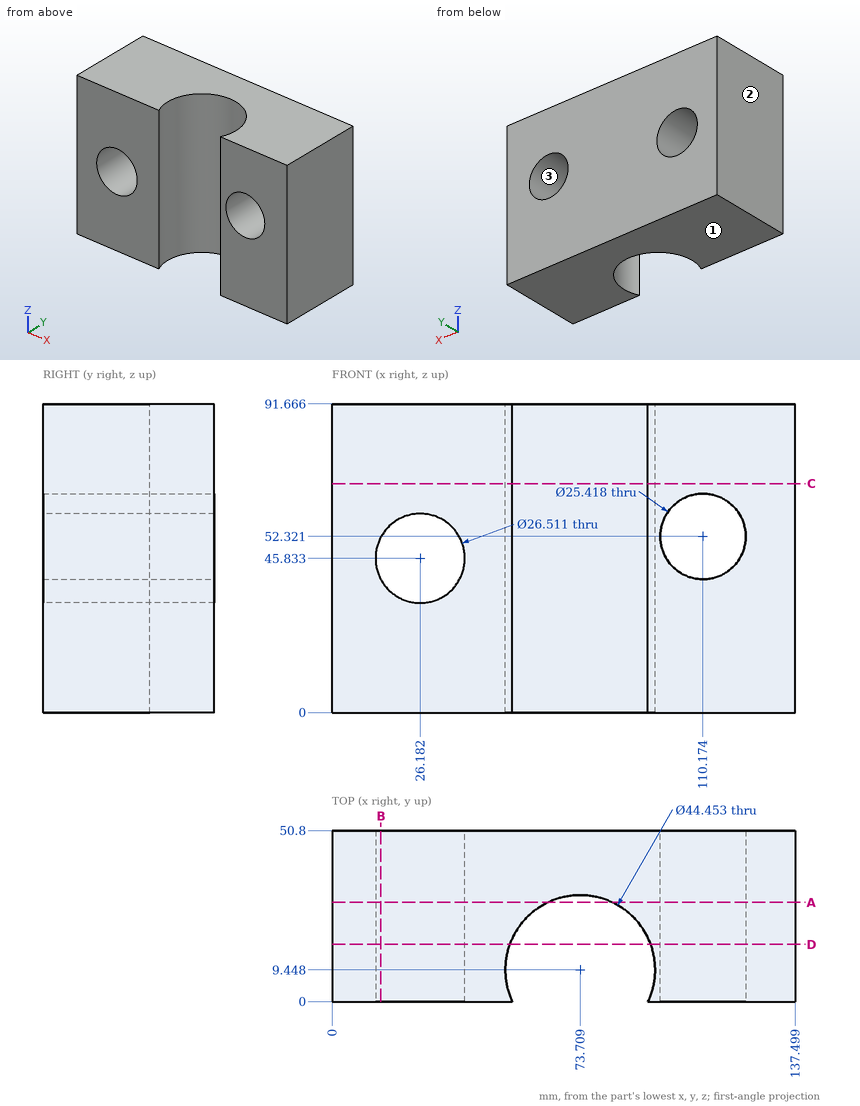
Study the drawing (mm; zero at the part's minimum x, y, z) and answer. Coordinates: 2 decimals unless noted, no trailing zeros. Loops run counter-clockwise (first coordinate to the right, second up) from the corner with the lowest first, then second, coordinate; pieces in that order, holes last. Notation, with made-up numbers: (18, 44.25) -> (30, 44.25) arc R27 ccw to (30, 77.25) -> close; hole circle Ø7 at (87.25, 89). An arc over 180 degrees is marked (long way). Answer in a Markdown table with one row per item. Add a question column.
1. The part is cut by section C-C, the plane z = 68. Write down the section's boundary in (x, y), then the cut area to 3 significant figures.
2. The part is cut by section A-A, the plane y = 29.5. Write down the section's boundary in (x, z) (1 decimal).
3. Flat-ended cylindrical pins translate along their axes: P1, Ø8, axis at x = 89.5, y = 33.5, coming from the -Z side; P2, Ø1, axis at x = 77.5, z = 80.5, coming from the -Y side; P3, Ø21, axis at x = 26.18, z = 45.83, coming from the +Y side; P4, Ø3, axis at x = 83.5, z = 29.5, coming from the -Y side (1 decimal). Find the tip coordinate at first contact, or state that the pin passes through.
4. Consider line 1 (X direction, y = 7, z = 62.5) (1 decimal); line 2 (Z direction, x = 104, y = 18) (1 decimal); line 3 (Z direction, x = 115.5, y = 13) (1 decimal). Determine where each line is inside the solid, lowest interval first. Write a range as [from, to].
5. The part is cut by section D-D, the plane y = 17. Write down the section's boundary in (x, z) (1 decimal).
6. The part is cut by section B-B, the plane x = 14.5. Write down the section's boundary in (y, z) (1 decimal), then the cut area to 3 significant figures.
7. Determine the mould class of the marked faces 1, 2 and 3 for opening direction Z: +Z half, -Z half, draft (parallel to the pull), parting line (faces both ways), or undercut.
Answer below:
| question | item | result |
|---|---|---|
| 1 | outline | (0, 0) -> (53.59, 0) arc R22.23 cw (long way) to (93.83, 0) -> (137.5, 0) -> (137.5, 50.8) -> (0, 50.8) -> close |
| 1 | area | 5,800 mm2 |
| 2 | outline | (0, 0) -> (64.1, 0) -> (64.1, 91.7) -> (0, 91.7) -> close; (83.3, 0) -> (137.5, 0) -> (137.5, 91.7) -> (83.3, 91.7) -> close; hole circle Ø26.5 at (26.2, 45.8); hole circle Ø25.4 at (110.2, 52.3) |
| 3 | P1 | z = 0 |
| 3 | P2 | y = 31.26 |
| 3 | P3 | through |
| 3 | P4 | y = 28.6 |
| 4 | line 1 | [0, 51.6], [95.8, 102.6], [117.8, 137.5] |
| 4 | line 2 | [0, 41.2], [63.4, 91.7] |
| 4 | line 3 | [0, 40.8], [63.9, 91.7] |
| 5 | outline | (0, 0) -> (52.8, 0) -> (52.8, 91.7) -> (0, 91.7) -> close; (94.6, 0) -> (137.5, 0) -> (137.5, 91.7) -> (94.6, 91.7) -> close; hole circle Ø26.5 at (26.2, 45.8); hole circle Ø25.4 at (110.2, 52.3) |
| 6 | outline | (0, 0) -> (50.8, 0) -> (50.8, 39.6) -> (0, 39.6) -> close; (0, 52.1) -> (50.8, 52.1) -> (50.8, 91.7) -> (0, 91.7) -> close |
| 6 | area | 4,020 mm2 |
| 7 | face 1 | -Z half |
| 7 | face 2 | draft |
| 7 | face 3 | undercut |
